```python
from build123d import *

# Parameters (mm, degrees)
F0_R     = 25
F1_DEPTH = 180
F2_SIZE2 = 5.3589838486
F2_SIZE  = 20
F4_D     = 17.5
F4_DEPTH = 60
F4_TIP   = 5.2575304165


with BuildPart() as f1:
    # F0 (on Top) → F1 (new body)
    with BuildSketch(Plane.XY):
        Circle(F0_R)
    extrude(amount=F1_DEPTH)

    # F2
    f2_edges = [f1.edges().sort_by_distance(p)[0] for p in [
        (-25, 0, 180),
    ]]
    f2_side = f1.faces().sort_by_distance((0, 0, 180))[0]
    chamfer(f2_edges, length=F2_SIZE, length2=F2_SIZE2, reference=f2_side)

    # F4
    with Locations(Plane(origin=(0, 0, 0), x_dir=(1, 0, 0), z_dir=(0, 0, -1))):
        with Locations((0, 0)):
            Hole(F4_D / 2, depth=F4_DEPTH)
            with Locations((0, 0, -(F4_DEPTH + F4_TIP / 2))):  # 118° drill point
                Cone(0, F4_D / 2, F4_TIP, mode=Mode.SUBTRACT)


solid = f1.part
```
Geometry check sheet. Reference: the model listing, model coordinates, mm. Coordinates: 2 decimals unless noted, no trailing zeros. Loops run counter-clockwise (first coordinate to the right, second up) from the corner with the lowest first, then second, coordinate; pieces in that order, holes last. Notation, with made-up numbers: (14.25, -21) - (49.25, -21) arc R21 ccw to (49.25, 11) - close; hole circle Ø7 at (45.5, 53). An arc over 180 degrees is marked (long way). One line per item, written item: value. Start each with the question number.
(1) Mould release check, pull along Y, two halves, no side actions. Record for faces 1 (the conical face through (-0.329, 1.483, 64.344)), 2 (the flat face through (0, 0, 180)), 3 (the conical face through (-1.355, -6.102, 179.665)), 4 (the cylindrical face through (6.944, 5.324, 30.42)): released by +Y, released by -Y, zero draft, split by the parting line, or undercut.
(2) Cross-section at A-A on z = 70. Enter the section's corners in (x, y).
(3) Depth check by flat-ended pin: P1, Ø12, axis at x = 14.5, z = 70, coming from the -Y side; P2, Ø6, axis at x = -6, y = 9.5, coming from the +Z side; P3, Ø3, axis at x = -18.5, z = 128.5, coming from the +Y side. Enter the tip coordinate at first touch or a pass-through.
(4) Material ranges on line 1 (Y direction, x = 0, z = 17.5); line 2 (Y direction, x = -1, z = 172.5); line 3 (X direction, y = 17, z = 143.5), recorded low to high. Write a range as [from, to].
Results below:
1. face 1: undercut
1. face 2: zero draft
1. face 3: split by the parting line
1. face 4: undercut
2. outline: circle Ø50 at (0, 0)
3. P1: stops at y = -23.51
3. P2: stops at z = 179.13
3. P3: stops at y = 18.33
4. line 1: y = [-25, -8.75], [8.75, 25]
4. line 2: y = [-24.98, 24.98]
4. line 3: x = [-18.33, 18.33]
